Source: CAD feature listing. Evaluate the final solid. Frame: model axes, mm. Face numbers are marked on the shaded views. A direction names the side the tool comes from. Give positions to 0.01 mm unless a question says otherwise; leave off trailing zeros. Order: outer loops, then holes, each group sorted by start corner. A loop starts at its lowest first (then second) coordinate and runs counter-clockwise, first axis right, second up.
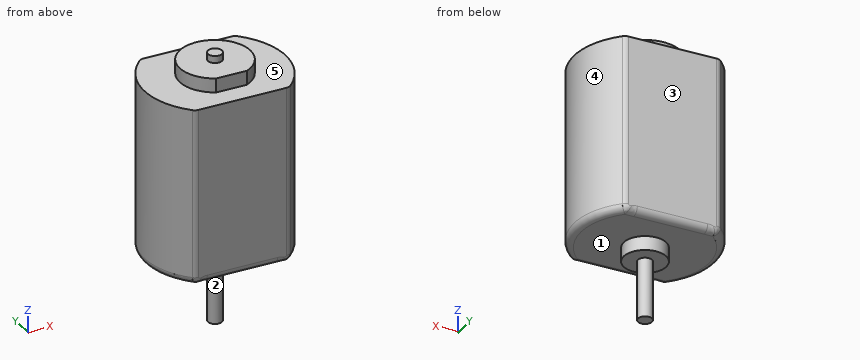
Autodesk Inventor part; units mm, degrees
ref_plane "YZ Plane" through (0, 0, 0) normal (1, 0, 0) x (0, 1, 0)
ref_plane "XZ Plane" through (0, 0, 0) normal (0, 1, 0) x (-1, 0, 0)
ref_plane "XY Plane" through (0, 0, 0) normal (0, 0, 1) x (1, 0, 0)
sketch "Sketch1" plane through (0, 0, 0) normal (0, 0, 1) x (1, 0, 0)
  circle A0 centre (0, 0) radius 1
  dimension "d0" = 2
extrude "Extrusion1" add sketch "Sketch1" along normal blind 8.4
sketch "Sketch2" plane through (0, 0, 8.4) normal (0, 0, 1) x (1, 0, 0)
  circle A0 centre (0, 0) radius 3
  dimension "d3" = 6
extrude "Extrusion2" add sketch "Sketch2" along normal blind 2
sketch "Sketch3" plane through (0, 0, 10.4) normal (0, 0, 1) x (1, 0, 0)
  line L0 (-6.6144, -7.5) -> (6.6144, -7.5)
  line L1 (6.6144, 7.5) -> (-6.6144, 7.5)
  line L2 (-10, -7.5) -> (10, 7.5) construction
  line L3 (10, -7.5) -> (-10, 7.5) construction
  arc A0 (-6.6144, 7.5) -> (-6.6144, -7.5) centre (0, 0) ccw
  arc A1 (6.6144, -7.5) -> (6.6144, 7.5) centre (0, 0) ccw
extrude "Extrusion3" add sketch "Sketch3" along normal blind 25
sketch "Sketch4" plane through (0, 0, 35.4) normal (0, 0, 1) x (1, 0, 0)
  arc A0 (2.1794, -4.5) -> (-2.1794, -4.5) centre (0, 0) ccw
  line L0 (0, -4.5) -> (2.1794, -4.5)
  line L1 (0, -4.5) -> (-2.1794, -4.5)
  dimension "d10" = 10
extrude "Extrusion4" add sketch "Sketch4" along normal blind 2
sketch "Sketch5" plane through (0, 0, 37.4) normal (0, 0, 1) x (1, 0, 0)
  circle A0 centre (0, 0) radius 1
  dimension "d14" = 2
extrude "Extrusion5" add sketch "Sketch5" along normal blind 1
fillet "Fillet7" radius 1 1 edges at (10, 0, 10.4)
fillet "Fillet8" radius 1 1 edges at (-10, 0, 10.4)
fillet "Fillet9" radius 1 5 edges at (0, -7.5, 10.4) (-6.0606, -7.5, 10.6339) (-6.6144, -7.5, 23.4) (6.0606, -7.5, 10.6339) (6.6144, -7.5, 23.4)
fillet "Fillet10" radius 1 5 edges at (0, 7.5, 10.4) (6.0606, 7.5, 10.6339) (6.6144, 7.5, 23.4) (-6.0606, 7.5, 10.6339) (-6.6144, 7.5, 23.4)
properties part number "motor" material "Aluminum 6061"
1) Section query D-D, the plane x = -3.5. Return the cut outline in (y, z).
Report:
outline: (-7.5, 11.4) arc R1 ccw to (-6.5, 10.4) - (6.5, 10.4) arc R1 ccw to (7.5, 11.4) - (7.5, 35.4) - (3.57, 35.4) - (3.57, 37.4) - (-3.57, 37.4) - (-3.57, 35.4) - (-7.5, 35.4) - close
2) Draft query along Y for the marked faces 1, 2 and 3. Return one class per face: +Y half, -Y half, draft (parallel to the pull), parting line (faces both ways), or undercut.
Report:
face 1: draft
face 2: parting line
face 3: +Y half
3) Section query C-C, the plane x = 0. Return the cut outline in (y, z), and give its area (3 significant figures).
Report:
outline: (-7.5, 11.4) arc R1 ccw to (-6.5, 10.4) - (-3, 10.4) - (-3, 8.4) - (-1, 8.4) - (-1, 0) - (1, 0) - (1, 8.4) - (3, 8.4) - (3, 10.4) - (6.5, 10.4) arc R1 ccw to (7.5, 11.4) - (7.5, 35.4) - (5, 35.4) - (5, 37.4) - (1, 37.4) - (1, 38.4) - (-1, 38.4) - (-1, 37.4) - (-4.5, 37.4) - (-4.5, 35.4) - (-7.5, 35.4) - close
area: 424 mm2
4) Section query A-A, the plane z = 33. Return the cut outline in (x, y), and give its area (3 significant figures).
Report:
outline: (-6.92, -7.22) arc R1 ccw to (-6.22, -7.5) - (6.22, -7.5) arc R1 ccw to (6.92, -7.22) arc R10 ccw to (6.92, 7.22) arc R1 ccw to (6.22, 7.5) - (-6.22, 7.5) arc R1 ccw to (-6.92, 7.22) arc R10 ccw to start
area: 269 mm2
5) Section query B-B, the plane y = 0. Return the cut outline in (x, z).
Report:
outline: (-10, 11.4) arc R1 ccw to (-9, 10.4) - (-3, 10.4) - (-3, 8.4) - (-1, 8.4) - (-1, 0) - (1, 0) - (1, 8.4) - (3, 8.4) - (3, 10.4) - (9, 10.4) arc R1 ccw to (10, 11.4) - (10, 35.4) - (5, 35.4) - (5, 37.4) - (1, 37.4) - (1, 38.4) - (-1, 38.4) - (-1, 37.4) - (-5, 37.4) - (-5, 35.4) - (-10, 35.4) - close
6) Reachability of the marked faces 4 and 5 from +Z, -Z, +X, -X, +Y, -Y: full face, straight path, thin tool, end or side. Return the list, or none.
Report:
face 4: +Z, -Z, +X
face 5: +Z
7) Pin query (flat end, axial travel): pin 1 (3 mm diameter, centred on y = -1, z = 8.5, fed in from -X); pin 2 (2 mm diameter, centred on x = 0.5, z = 8.5, fed in from -Y); pin 3 (1.5 mm diameter, centred on x = -7.5, y = -4.5, fed in from -Z). Return the tip coordinate at first contact, or that it passes through.
Report:
pin 1: stops at x = -3
pin 2: stops at y = -3
pin 3: stops at z = 10.4
8) Material intervals for L1, parallel to Z at x = 1.5, y = -6.5; L2, parallel to Z at x = -3.75, y = -3; L3, parallel to X at y = 4.75, z = 33.5, sorted ascending.
Report:
L1: z = 10.4 to 35.4
L2: z = 10.4 to 37.4
L3: x = -8.8 to 8.8
